Build history of the part. All positions in model axes, mm. Coordinates: 2 decimals unless noted, no trailing zeros. Loops run counter-clockwise (first coordinate to the right, second up) from the corner with the lowest first, then second, coordinate; pieces in that order, holes last. Notation, with made-up numbers: (0, -4.5) - (49, -4.5) arc R13 ccw to (49, 4.5) - close; hole circle Ø11 at (-17, -1.75). An arc over 180 degrees is marked (long way). One line per item, written item: value.
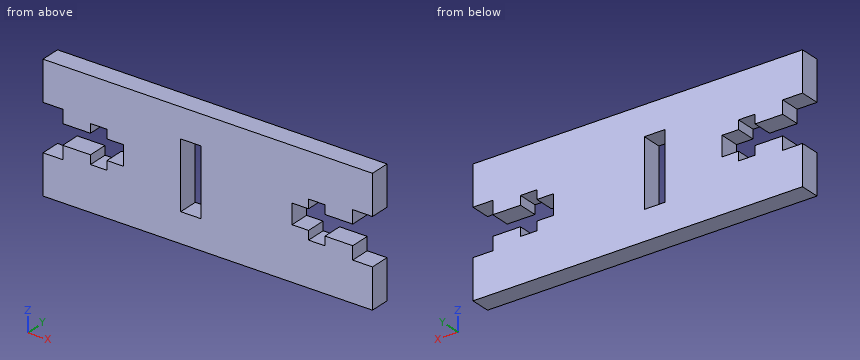
```python
from build123d import *

# Parameters (mm, degrees)
SKETCH2_W           = 50
SKETCH2_H           = 19
BOSS_EXTRUDE1_DEPTH = 3
CUT_EXTRUDE1_DEPTH  = 4
SKETCH4_W           = 3.1
SKETCH4_H           = 10.1
CUT_EXTRUDE2_DEPTH  = 4


with BuildPart() as part:
    # Sketch2 → Boss-Extrude1 (new body)
    with BuildSketch(Plane(origin=(0, 0, 0), x_dir=(1, 0, 0), z_dir=(0, 1, 0))):
        with Locations((25, 9.5)):
            Rectangle(SKETCH2_W, SKETCH2_H)
    extrude(amount=BOSS_EXTRUDE1_DEPTH)

    # Sketch3 → Cut-Extrude1 (cut, through all)
    with BuildSketch(Plane(origin=(0, 3, 0), x_dir=(1, 0, 0), z_dir=(0, 1, 0))):
        Polygon((0, 13), (3, 13), (3, 11), (7.2, 11), (7.2, 12.35), (9.7, 12.35), (9.7, 11), (12.2, 11), (12.2, 8), (9.7, 8), (9.7, 6.65), (7.2, 6.65), (7.2, 8), (3, 8), (3, 6), (0, 6), align=None)
    cut_extrude1 = extrude(amount=-CUT_EXTRUDE1_DEPTH, mode=Mode.SUBTRACT)

    # Mirror1: Cut-Extrude1 across plane
    add(cut_extrude1.mirror(Plane(origin=(25, 0, 0), x_dir=(0, 0, 1), z_dir=(1, 0, 0))), mode=Mode.SUBTRACT)

    # Sketch4 → Cut-Extrude2 (cut, through all)
    with BuildSketch(Plane(origin=(0, 3, 0), x_dir=(1, 0, 0), z_dir=(0, 1, 0))):
        with Locations((22.45, 9.5)):
            Rectangle(SKETCH4_W, SKETCH4_H)
    extrude(amount=-CUT_EXTRUDE2_DEPTH, mode=Mode.SUBTRACT)


solid = part.part
```
Item 1: Probe probe 1 along X at (y, z) = (0.35, -5.75); probe 2 along Z at (x, y) = (21.5, 0.8); probe 3 along Z at (x, y) = (45.5, 2.1). List the from-to ranges inside material, lowest first. Write a range as from..to.
Check result:
probe 1: x = 0..20.9, 24..50
probe 2: z = -19..-14.55, -4.45..0
probe 3: z = -19..-11, -8..0
Item 2: Cut at A-A, the plane x = 41.5. Write the cut outline in (y, z).
Check result:
outline: (0, -19) - (3, -19) - (3, -12.35) - (0, -12.35) - close; (0, -6.65) - (3, -6.65) - (3, 0) - (0, 0) - close
Item 3: Drop flat-ended pins along their axis: P1, Ø1.5, axis at y = 1, z = -12, coming from the -X side; P2, Ø0.7, axis at y = 2, z = -11.5, coming from the +X side; P3, Ø1.5, axis at y = 1, z = -9, coming from the -X side. Give the stop position or say it passes through.
Check result:
P1: stops at x = 3
P2: stops at x = 47
P3: stops at x = 12.2
Item 4: Cut at B-B, the plane x = 22. Write the cut outline in (y, z).
Check result:
outline: (0, -19) - (3, -19) - (3, -14.55) - (0, -14.55) - close; (0, -4.45) - (3, -4.45) - (3, 0) - (0, 0) - close
